Work out the finished part from the listing and answer in its coordinate system (mm). A direction names the side the tool comes from. Round coordinates to 2 decimals unless told otherwise and drop trailing zeros. Write each loop counter-clockwise with the first axis right and the second up, starting at its lowest first coordinate (ties: lowest second). Pieces come first, ordered by that corner, then holes. Notation, with made-up numbers: (79.25, 5.5) -> (122.25, 5.5) arc R12 ccw to (122.25, 18.5) -> close; hole circle Ø4 at (36.5, 77). An arc over 180 degrees is marked (long way). One line per item, written item: value.
```python
from build123d import *

# Parameters (mm, degrees)
F1_DEPTH      = 30.15
F1_DEPTH_BACK = 30.15
F2_R          = 3.5
F3_DEPTH      = 25
F4_START      = 3
F2_R_2        = 5
F4_DEPTH      = 22
F5_R          = 3.5
F6_DEPTH      = 25
F7_START      = 3
F5_R_2        = 5
F7_DEPTH      = 22


with BuildPart() as f1:
    # F0 (on Right) → F1 (new body, two sides)
    with BuildSketch(Plane.YZ) as f1_sk:
        Polygon((-39.15, 0), (0, 0), (0, 39.15), align=None)
    extrude(amount=F1_DEPTH)
    extrude(f1_sk.sketch, amount=-F1_DEPTH_BACK)

    # F2 (on Front) → F3 (cut)
    with BuildSketch(Plane.XZ):
        with Locations((-20, 29.3)):
            Circle(F2_R)
        with Locations((0, 29.3)):
            Circle(F2_R)
        with Locations((20, 29.3)):
            Circle(F2_R)
    extrude(amount=F3_DEPTH, mode=Mode.SUBTRACT)

    # F2 (on Front) → F4 (cut)
    with BuildSketch(Plane.XZ.offset(F4_START)):
        with Locations((20, 29.3)):
            Circle(F2_R_2)
        with Locations((20, 29.3)):
            Circle(F2_R, mode=Mode.SUBTRACT)
        with Locations((0, 29.3)):
            Circle(F2_R_2)
        with Locations((0, 29.3)):
            Circle(F2_R, mode=Mode.SUBTRACT)
        with Locations((-20, 29.3)):
            Circle(F2_R_2)
        with Locations((-20, 29.3)):
            Circle(F2_R, mode=Mode.SUBTRACT)
    extrude(amount=F4_DEPTH, mode=Mode.SUBTRACT)

    # F5 (on Top) → F6 (cut)
    with BuildSketch(Plane.XY):
        with Locations((20, -29.3)):
            Circle(F5_R)
        with Locations((0, -29.3)):
            Circle(F5_R)
        with Locations((-20, -29.3)):
            Circle(F5_R)
    extrude(amount=F6_DEPTH, mode=Mode.SUBTRACT)

    # F5 (on Top) → F7 (cut)
    with BuildSketch(Plane.XY.offset(F7_START)):
        with Locations((-20, -29.3)):
            Circle(F5_R_2)
        with Locations((-20, -29.3)):
            Circle(F5_R, mode=Mode.SUBTRACT)
        with Locations((0, -29.3)):
            Circle(F5_R_2)
        with Locations((0, -29.3)):
            Circle(F5_R, mode=Mode.SUBTRACT)
        with Locations((20, -29.3)):
            Circle(F5_R_2)
        with Locations((20, -29.3)):
            Circle(F5_R, mode=Mode.SUBTRACT)
    extrude(amount=F7_DEPTH, mode=Mode.SUBTRACT)


solid = f1.part
```
(1) Consider probe 1 along X at (y, z) = (-29, 8); probe 2 along Z at (x, y) = (0, -1.55); probe 3 along Z at (x, y) = (-20, -8.25). Determine where each line is inside the solid, lowest interval first.
Reported:
probe 1: x = -30.15 to -24.99, -15.01 to -4.99, 4.99 to 15.01, 24.99 to 30.15
probe 2: z = 0 to 25.8, 32.8 to 37.6
probe 3: z = 0 to 24.3
(2) For a pull along X with two mould halves and no side action, classify faces 1 (the face through (21, -3, 33)), 2 (the face through (-30.15, -11, 11)), 3 (the face through (30.15, -11, 11)) as pulls with the +X half, pulls with the -X half, needs draft (parallel to the pull), parting line crosses it, or undercut.
Reported:
face 1: undercut
face 2: pulls with the -X half
face 3: pulls with the +X half
(3) Flat-ended cylindrical pins translate along their axes: pin 1 Ø3 at (x, z) = (1, 31.5) entering from -Y; pin 2 Ø1 at (x, y) = (14.5, -11) entering from +Z; pin 3 Ø11 at (x, z) = (20, 29.3) entering from -Y. Find the tip coordinate at first contact, or state that the pin passes through.
Reported:
pin 1: stops at y = -3
pin 2: stops at z = 28.65
pin 3: stops at y = -15.35
(4) Find section B-B on x = -20. Give the vertices of the cut face in (y, z).
Reported:
outline: (-39.15, 0) -> (-32.8, 0) -> (-32.8, 3) -> (-34.3, 3) -> (-34.3, 4.85) -> close; (-25.8, 0) -> (0, 0) -> (0, 25.8) -> (-3, 25.8) -> (-3, 24.3) -> (-14.85, 24.3) -> (-24.3, 14.85) -> (-24.3, 3) -> (-25.8, 3) -> close; (-4.85, 34.3) -> (-3, 34.3) -> (-3, 32.8) -> (0, 32.8) -> (0, 39.15) -> close
(5) Find section A-A on y = -29.3. Give the vertices of the cut face in (x, z), plus the area to 3 significant figures.
Reported:
outline: (-30.15, 0) -> (-23.5, 0) -> (-23.5, 3) -> (-25, 3) -> (-25, 9.85) -> (-30.15, 9.85) -> close; (-16.5, 0) -> (-3.5, 0) -> (-3.5, 3) -> (-5, 3) -> (-5, 9.85) -> (-15, 9.85) -> (-15, 3) -> (-16.5, 3) -> close; (3.5, 0) -> (16.5, 0) -> (16.5, 3) -> (15, 3) -> (15, 9.85) -> (5, 9.85) -> (5, 3) -> (3.5, 3) -> close; (23.5, 0) -> (30.15, 0) -> (30.15, 9.85) -> (25, 9.85) -> (25, 3) -> (23.5, 3) -> close
area: 325 mm2
(6) Find section C-C on x = -8.5. Give the vertices of the cut face in (y, z), plus the area to 3 significant figures.
Reported:
outline: (-39.15, 0) -> (0, 0) -> (0, 39.15) -> close
area: 766 mm2
(7) Find section D-D on y = -33.5. Give the vertices of the cut face in (x, z).
Reported:
outline: (-30.15, 0) -> (30.15, 0) -> (30.15, 5.65) -> (22.71, 5.65) -> (22.71, 3) -> (17.29, 3) -> (17.29, 5.65) -> (2.71, 5.65) -> (2.71, 3) -> (-2.71, 3) -> (-2.71, 5.65) -> (-17.29, 5.65) -> (-17.29, 3) -> (-22.71, 3) -> (-22.71, 5.65) -> (-30.15, 5.65) -> close
(8) A tool of negligible diameter and unlimited length cuts with its end or side. For faces 4 (the face through (-1.08, -7.57, 24.42)), 5 (the face through (0.42, -19.3, 19.85)), 6 (the face through (-20.651, -24.343, 7.525)), from which of +Z, -Z, +X, -X, +Y, -Y can it reach the whole face along a straight path? Write none if from no direction.
Reported:
face 4: -Y
face 5: +Z, +X, -X, -Y
face 6: +Z
